Work out the finished part from the listing and answer in its coordinate system (mm). A direction names the side the tool comes from. Give positions to 0.01 mm unless a question says otherwise; leave off trailing zeros. Write each loop counter-clockwise with the first axis right and the second up, starting at its lowest first coordinate (ties: lowest second). Pieces come first, ordered by that corner, then holes. Notation, with made-up numbers: (74.25, 16.25) -> (130.25, 16.25) arc R25 cw to (130.25, 51.25) -> close; hole circle Ø4 at (85, -28). An arc over 180 degrees is marked (long way). Use a Markdown table: item, result. Add a question column.
Q1. Section D-D, the plane y = 2.5 is taken. Give the vertices of the cut face in (x, z), plus the area to 3 significant figures.
Q2. Section A-A, the plane x = 12.75 is taken. Give the vertices of the cut face in (y, z), plus the area to 3 significant figures.
Q3. For a pull along Z with two mould halves and no side action, classify faces 1 (the face through (8, 0, 5)), 2 (the face through (8, 11.4, 4)), 3 (the face through (8, 6, 10.7)) as pulls with the +Z half, pulls with the -Z half, needs draft (parallel to the pull), parting line crosses it, or undercut.
Q4. Section B-B, the plane z = 6.25 is taken. Give the vertices of the cut face in (x, y).
Q5. For faces 4 (the face through (0, 6, 5)), 5 (the face through (8, 6, 3.8)), determine the directions among +Z, -Z, +X, -X, +Y, -Y from which every point of the face is accessible in a straight line to the end or side of a thin tool.
Q6. Consider line 1 (Y direction, x = 7, z = 5.25); line 2 (Z direction, x = 6, y = 4); line 3 (Z direction, x = 8.5, y = 9.25). Determine where each line is inside the solid, lowest interval first.
Q7. Section C-C, the plane y = 4 is taken. Give the vertices of the cut face in (x, z), plus the area to 3 significant figures.
from build123d import *

# Parameters (mm, degrees)
F0_W     = 16.4
F0_H     = 12.4
F1_DEPTH = 10.7
F2_T     = -1
F3_W     = 5.4
F3_H     = 3.1
F4_DEPTH = 15.4
F5_SIZE  = 2


with BuildPart() as f1:
    # F0 (on Top) → F1 (new body)
    with BuildSketch(Plane.XY):
        with Locations((8.2, 6.2)):
            Rectangle(F0_W, F0_H)
    extrude(amount=F1_DEPTH)

    # F2
    f2_openings = [f1.faces().sort_by_distance(p)[0] for p in [
        (0, 6.2, 5.35),
    ]]
    offset(amount=F2_T, openings=f2_openings)

    # F3 (on face) → F4 (join, through all)
    with BuildSketch(Plane(origin=(0, 0, 0), x_dir=(0, -1, 0), z_dir=(-1, 0, 0))):
        with Locations((-6.2, 5.35)):
            Rectangle(F3_W, F3_H)
    extrude(amount=-F4_DEPTH)

    # F5
    f5_edges = [f1.edges().sort_by_distance(p)[0] for p in [
        (7.7, 11.4, 9.7),
        (7.7, 1, 9.7),
    ]]
    chamfer(f5_edges, length=F5_SIZE)


solid = f1.part
Result set:
| question | item | result |
|---|---|---|
| 1 | outline | (0, 0) -> (16.4, 0) -> (16.4, 10.7) -> (0, 10.7) -> (0, 9.2) -> (15.4, 9.2) -> (15.4, 1) -> (0, 1) -> close |
| 1 | area | 49.2 mm2 |
| 2 | outline | (0, 0) -> (12.4, 0) -> (12.4, 10.7) -> (0, 10.7) -> close; (3.5, 3.8) -> (8.9, 3.8) -> (8.9, 6.9) -> (3.5, 6.9) -> close; hole (1, 1) -> (11.4, 1) -> (11.4, 7.7) -> (9.4, 9.7) -> (3, 9.7) -> (1, 7.7) -> close |
| 2 | area | 62.9 mm2 |
| 3 | face 1 | needs draft |
| 3 | face 2 | undercut |
| 3 | face 3 | pulls with the +Z half |
| 4 | outline | (0, 0) -> (16.4, 0) -> (16.4, 12.4) -> (0, 12.4) -> (0, 11.4) -> (15.4, 11.4) -> (15.4, 8.9) -> (0, 8.9) -> (0, 3.5) -> (15.4, 3.5) -> (15.4, 1) -> (0, 1) -> close |
| 5 | face 4 | +Z, -Z, -X, +Y, -Y |
| 5 | face 5 | -X |
| 6 | line 1 | y = 0 to 1, 3.5 to 8.9, 11.4 to 12.4 |
| 6 | line 2 | z = 0 to 1, 3.8 to 6.9, 9.7 to 10.7 |
| 6 | line 3 | z = 0 to 1, 9.7 to 10.7 |
| 7 | outline | (0, 0) -> (16.4, 0) -> (16.4, 10.7) -> (0, 10.7) -> (0, 9.7) -> (15.4, 9.7) -> (15.4, 6.9) -> (0, 6.9) -> (0, 3.8) -> (15.4, 3.8) -> (15.4, 1) -> (0, 1) -> close |
| 7 | area | 89.2 mm2 |
